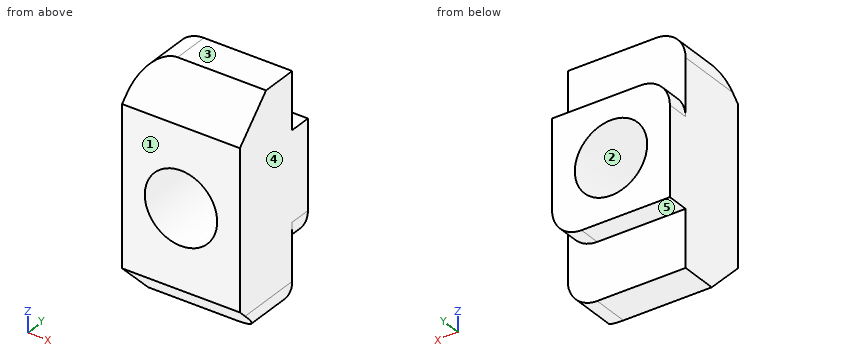
```python
from build123d import *

# Parameters (mm, degrees)
BOSS_EXTRUDE1_DEPTH = 4
FILLET1_R           = 2
TAP1_D              = 4.917


with BuildPart() as part:
    # Sketch1 → Boss-Extrude1 (new, symmetric)
    with BuildSketch(Plane(origin=(0, 0, 0), x_dir=(0, 0, -1), z_dir=(1, 0, 0))):
        Polygon((-4, 0), (4, 0), (4, -1.5), (7.85, -1.5), (7.85, -4), (5.35, -6.5), (-5.35, -6.5), (-7.85, -4), (-7.85, -1.5), (-4, -1.5), align=None)
    extrude(amount=BOSS_EXTRUDE1_DEPTH, both=True)

    # Fillet1
    fillet1_edges = [part.edges().sort_by_distance(p)[0] for p in [
        (-4, -2.75, 7.85),
        (-4, -0.75, 4),
        (4, -2.75, -7.85),
        (4, -0.75, -4),
    ]]
    fillet(fillet1_edges, radius=FILLET1_R)

    # Tap1 (through all)
    with Locations(Plane(origin=(0, 0, 0), x_dir=(1, 0, 0), z_dir=(0, 1, 0))):
        with Locations((0, 0)):
            Hole(TAP1_D / 2)


solid = part.part
```
The model under review builds one solid part; all positions refer to its coordinate system, in mm. Face numbers are marked on the shaded views. A direction names the side the tool comes from. Coordinates: 2 decimals unless noted, no trailing zeros. Write each loop counter-clockwise with the first axis right and the second up, starting at its lowest first coordinate (ties: lowest second). Pieces come first, ordered by that corner, then holes. Notation, with made-up numbers: (-13.5, 78.5) - (17.5, 78.5) arc R11 cw to (17.5, 85.5) - close; hole circle Ø8 at (38, 29). An arc over 180 degrees is marked (long way). Answer in a Markdown table with one row per item. Add a question column.
Q1. Consider section B-B on z = 0. Give the boundary of the cut face in (x, y).
Q2. Consider section A-A on y = -1.25. Give the boundary of the cut face in (x, z), then the cut area to 3 significant figures.
Q3. For the marked faces 4 and 5, list the 3-axis set-ups (+Z, -Z, +X, -X, +Y, -Y) from which the entire face can be reached by the end or side of a thin tool; tool diameter is ignored.
Q4. Consider section D-D on y = -3.5. Give the boundary of the cut face in (x, z), then the cut area to 3 significant figures.
Q5. Draft analysis for pull direction Z (two halves, no side actions). For the marked faces 1, 2 and 3, state which applies: +Z half, -Z half, draft (parallel to the pull), parting line (faces both ways), or undercut.
Q6. Consider section C-C on x = 0. Give the boundary of the cut face in (y, z).
Q7. To check wall thickness, follow line 1 along Z through (x, y) = (0, -3.25); line 2 along X through (y, z) = (-4.5, -1.5); line 3 along Y through (x, z) = (1.5, -5). State the ranges of each line that lie inside material, in increasing order. Write a range as from..to.
Answers below:
| question | item | result |
|---|---|---|
| 1 | outline | (-4, -6.5) - (-2.46, -6.5) - (-2.46, 0) - (-4, 0) - close; (2.46, -6.5) - (4, -6.5) - (4, 0) - (2.46, 0) - close |
| 2 | outline | (-4, -4) - (2, -4) arc R2 ccw to (4, -2) - (4, 4) - (-2, 4) arc R2 ccw to (-4, 2) - close; hole circle Ø4.92 at (0, 0) |
| 2 | area | 43.3 mm² |
| 3 | face 4 | +Z, -Z, +X, +Y, -Y |
| 3 | face 5 | -Z, +X, -X, +Y |
| 4 | outline | (-4, -7.85) - (2, -7.85) arc R2 ccw to (4, -5.85) - (4, 7.85) - (-2, 7.85) arc R2 ccw to (-4, 5.85) - close; hole circle Ø4.92 at (0, 0) |
| 4 | area | 105 mm² |
| 5 | face 1 | draft |
| 5 | face 2 | undercut |
| 5 | face 3 | +Z half |
| 6 | outline | (-6.5, -5.35) - (-4, -7.85) - (-1.5, -7.85) - (-1.5, -4) - (0, -4) - (0, -2.46) - (-6.5, -2.46) - close; (-6.5, 2.46) - (0, 2.46) - (0, 4) - (-1.5, 4) - (-1.5, 7.85) - (-4, 7.85) - (-6.5, 5.35) - close |
| 7 | line 1 | -7.85..-2.46, 2.46..7.85 |
| 7 | line 2 | -4..-1.95, 1.95..4 |
| 7 | line 3 | -6.5..-1.5 |
